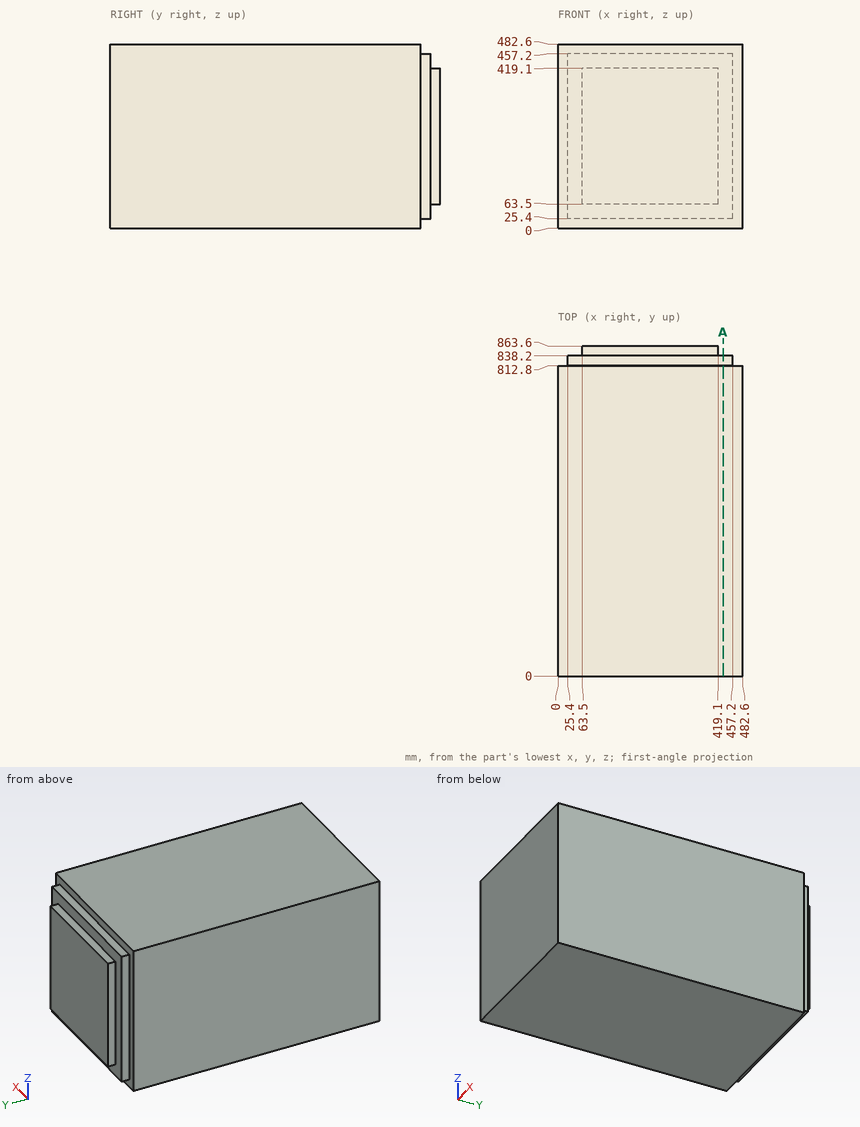
Geometry check sheet. Reference: drawing and pictorial views, mm from the part's lowest x, y, z. Round coordinates to 2 decimals unless told otherwise and drop trailing zeros. Write each loop counter-clockwise with the first axis right and the second up, starting at its lowest first coordinate (ties: lowest second). Pieces come first, ordered by that corner, then holes.
1. Gauge pin test, flat ends, axial feed: P1, Ø20.5, axis at y = 825, z = 206.5, coming from the -X side; P2, Ø7.5, axis at y = 847.5, z = 182, coming from the +X side; P3, Ø7.5, axis at x = 217.5, y = 846, coming from the -Z side. Record the tip position at first contact, or that the pin passes through.
2. Scan lines: L1, parallel to Y at x = 423, z = 420.5; L2, parallel to Z at x = 261, y = 824.5. Record each from-to range of solid material in increasing order.
3. Section check A-A on x = 432. Enter the section's corners in (y, z).
Answer:
1. P1: stops at x = 25.4
1. P2: stops at x = 419.1
1. P3: stops at z = 63.5
2. L1: y = 0 to 838.2
2. L2: z = 25.4 to 457.2
3. outline: (0, 0) - (812.8, 0) - (812.8, 25.4) - (838.2, 25.4) - (838.2, 457.2) - (812.8, 457.2) - (812.8, 482.6) - (0, 482.6) - close
